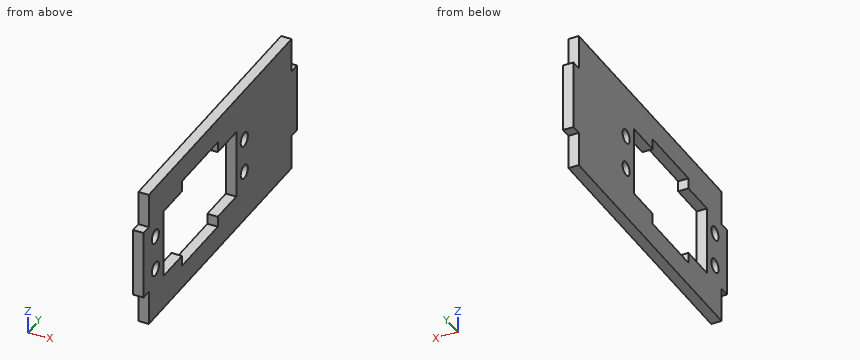
from build123d import *

# Parameters (mm, degrees)
BOSS_EXTRU_1_DEPTH      = 3
ESQUISSE2_R             = 2
ENL_V_MAT_EXTRU_1_DEPTH = 99.4971691


with BuildPart() as part:
    # Esquisse1 → Boss.-Extru.1 (new body)
    with BuildSketch(Plane(origin=(3, 0, 0), x_dir=(0, 0, -1), z_dir=(1, 0, 0))):
        Polygon((-31.50377455, 89.275579073), (-31.50377455, 86.275579073), (-41.50377455, 86.275579073), (-41.50377455, 6.275579073), (-31.50377455, 6.275579073), (-31.50377455, 3.275579073), (-11.50377455, 3.275579073), (-11.50377455, 6.275579073), (-1.50377455, 6.275579073), (-1.50377455, 86.275579073), (-11.50377455, 86.275579073), (-11.50377455, 89.275579073), align=None)
    extrude(amount=-BOSS_EXTRU_1_DEPTH)

    # Esquisse2 → Enlèv. mat.-Extru.1 (cut, through all)
    with BuildSketch(Plane.ZY):
        with Locations(Location((26.40377455, 9.975579073, 0), (0, 0, 180))):
            Circle(ESQUISSE2_R)
        with Locations(Location((16.40377455, 59.775579073, 0), (0, 0, 180))):
            Circle(ESQUISSE2_R)
        with Locations(Location((26.40377455, 59.775579073, 0), (0, 0, 180))):
            Circle(ESQUISSE2_R)
        with Locations(Location((16.40377455, 9.975579073, 0), (0, 0, 180))):
            Circle(ESQUISSE2_R)
        Polygon((11.40377455, 44.925579073), (11.40377455, 55.275579073), (31.40377455, 55.275579073), (31.40377455, 44.925579073), (34.50377455, 44.925579073), (34.50377455, 24.825579073), (31.40377455, 24.825579073), (31.40377455, 14.475579073), (11.40377455, 14.475579073), (11.40377455, 24.825579073), (8.30377455, 24.825579073), (8.30377455, 44.925579073), align=None)
    extrude(amount=-ENL_V_MAT_EXTRU_1_DEPTH, mode=Mode.SUBTRACT)


solid = part.part
The listing builds one solid part. Answer for the finished solid, in the listing's coordinates (mm). Round coordinates to 2 decimals unless told otherwise and drop trailing zeros. Order: outer loops, then holes, each group sorted by start corner. A loop starts at its lowest first (then second) coordinate and runs counter-clockwise, first axis right, second up. Notation, with made-up numbers: M -38,-14.5 L 1,-14.5 A13 ccw 1,-8.5 Z; hole C -35.5,-18.75 d2. An arc over 180 degrees is marked long. Answer in a Markdown table with one row per item. Add a question column.
1) The part is cut by section A-A on y = 39.5. Determine the outline of the cut face in (x, z).
2) The part is cut by section C-C on y = 61. Determine the outline of the cut face in (x, z).
3) The part is cut by section B-B on z = 22. Determine the outline of the cut face in (x, y), plus the area to 3 significant figures.
4) Flat-ended cylindrical pins translate along their axes: pin 1 Ø0.9 at (x, z) = (2, 5) entering from -Y; pin 2 Ø0.9 at (x, y) = (2, 88) entering from +Z; pin 3 Ø8 at (y, z) = (24, 18.5) entering from -X. Find the tip coordinate at first contact, or state that the pin passes through.
5) Consider line 1 along Y through (x, z) = (1.2, 29.5); line 2 along Z through (x, y) = (1.25, 50); line 3 along Y through (x, z) = (2.35, 18). Determine where each line is inside the solid, lowest interval first. Write a range as from..to.
6) The part is cut by section D-D on x = 1.8. Determine the outline of the cut face in (y, z).
Findings below:
| question | item | result |
|---|---|---|
| 1 | outline | M 0,1.5 L 3,1.5 L 3,8.3 L 0,8.3 Z; M 0,34.5 L 3,34.5 L 3,41.5 L 0,41.5 Z |
| 2 | outline | M 0,1.5 L 3,1.5 L 3,14.82 L 0,14.82 Z; M 0,17.99 L 3,17.99 L 3,24.82 L 0,24.82 Z; M 0,27.99 L 3,27.99 L 3,41.5 L 0,41.5 Z |
| 3 | outline | M 0,3.28 L 3,3.28 L 3,14.48 L 0,14.48 Z; M 0,55.28 L 3,55.28 L 3,89.28 L 0,89.28 Z |
| 3 | area | 136 mm² |
| 4 | pin 1 | stops at y = 6.28 |
| 4 | pin 2 | stops at z = 31.5 |
| 4 | pin 3 | passes through |
| 5 | line 1 | y = 3.28..14.48, 55.28..89.28 |
| 5 | line 2 | z = 1.5..11.4, 31.4..41.5 |
| 5 | line 3 | y = 3.28..8.77, 11.18..14.48, 55.28..58.57, 60.98..89.28 |
| 6 | outline | M 3.28,11.5 L 6.28,11.5 L 6.28,1.5 L 86.28,1.5 L 86.28,11.5 L 89.28,11.5 L 89.28,31.5 L 86.28,31.5 L 86.28,41.5 L 6.28,41.5 L 6.28,31.5 L 3.28,31.5 Z; hole C 9.98,16.4 d4; hole C 9.98,26.4 d4; hole M 14.48,11.4 L 24.83,11.4 L 24.83,8.3 L 44.93,8.3 L 44.93,11.4 L 55.28,11.4 L 55.28,31.4 L 44.93,31.4 L 44.93,34.5 L 24.83,34.5 L 24.83,31.4 L 14.48,31.4 Z; hole C 59.78,16.4 d4; hole C 59.78,26.4 d4 |
